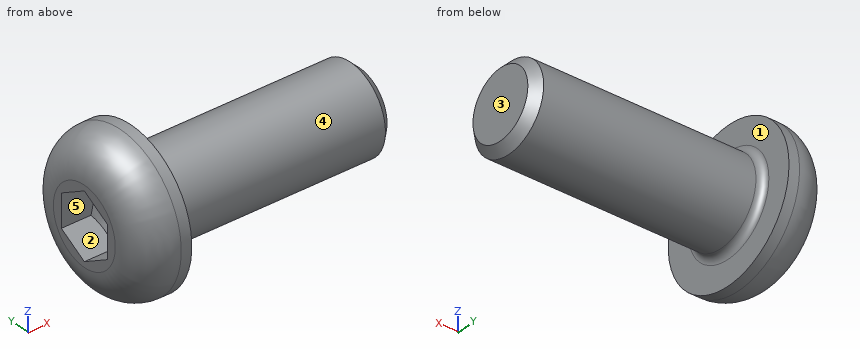
Autodesk Inventor part; units mm, degrees
ref_plane "Work Plane1" through (29, 0, 0) normal (0, -1, 0) x (1, 0, 0)
ref_plane "YZ Plane" through (0, 0, 0) normal (1, 0, 0) x (0, 1, 0)
ref_plane "XZ Plane" through (0, 0, 0) normal (0, 1, 0) x (-1, 0, 0)
sketch "Sketch1" plane through (0, 0, 0) normal (0, 0, 1) x (1, 0, 0)
  line L0 (0.1133, 0) -> (16, 0)
  line L1 (16, 0) -> (16, 3)
  line L2 (16, 3) -> (3, 3)
  line L3 (3, 3) -> (2.3864, 3)
  line L4 (2.3864, 3) -> (0, 3)
  line L5 (0, 3) -> (0, 5.25)
  line L6 (0, 5.25) -> (-3.3, 5.25)
  line L7 (-3.3, 5.25) -> (-3.3, 2.3094)
  line L8 (-3.3, 2.3094) -> (-1.22, 2.3094)
  line L9 (-1.22, 2.3094) -> (0.1133, 0)
  line L10 (-7.16, 0) -> (19.86, 0)
  line L11 (0, -1.05) -> (0, 6.3)
  line L12 (3, 3) -> (0, 3) construction
  dimension "d1" = 13
  dimension "d2" = 0.6136
  dimension "d3" = 3.3
  dimension "d4" = 2.08
  dimension "d5" = 60
  dimension "d6" = 6
  dimension "d7" = 6
  dimension "d8" = 4.6188
  dimension "d9" = 10.5
  dimension "d26" = 16
revolve "Body" add sketch "Sketch1" angle 360 about axis through (0.1133, 0, 0) along (1, 0, 0) contours L9 L11 L4 L3 L2 L1 L0 | L9 L8 L7 L6 L5 L11
sketch "Sketch2" plane through (-3.3, 0, 0) normal (-1, 0, 0) x (0, 0, 1)
  circle A0 centre (0, 0) radius 2.3094
  line L0 (0, -7.35) -> (0, 7.35)
  line L1 (-7.35, 0) -> (7.35, 0)
  line L2 (2.3094, 0) -> (1.1547, -2)
  line L3 (1.1547, -2) -> (-1.1547, -2)
  line L4 (-1.1547, -2) -> (-2.3094, 0)
  line L5 (-2.3094, 0) -> (-1.1547, 2)
  line L6 (-1.1547, 2) -> (1.1547, 2)
  line L7 (1.1547, 2) -> (2.3094, 0)
extrude "Slot" add sketch "Sketch2" against normal up to next contours L7 A0 | A0 L2 | L6 L0 A0 | A0 L0 L3 | L0 L6 A0 | A0 L3 L0 | L4 A0 | A0 L5
fillet "Fillet1" radius 2.56 1 edges at (-3.3, -5.25, 0)
thread "Thread"
chamfer "Chamfer1" distance 0.6135 distance2 0.6135 1 edges at (16, -3, 0) measured on face at (16, -1.1424, 0.935)
ref_plane "Work Plane1" through (29, 0, 0) normal (0, -1, 0) x (1, 0, 0)
fillet "Fillet2" radius 0.5 1 edges at (0, -3, 0)
equation "\"d1\" = GEL"
equation "\"d3\" = KOH"
equation "\"d4\" = INTI"
equation "\"d6\" = GD"
equation "\"d7\" = BDM"
equation "\"d8\" = 1.1547 * SW"
equation "\"d9\" = KOD"
equation "\"d26\" = NLG"
equation "\"d30\" = R"
equation "\"d17\" = RR"
equation "\"d13\" = GEL"
equation "\"d15\" = -0.5 * SPD + 0.5 * GD"
equation "\"d16\" = GUL"
equation "\"GD\" = NND"
equation "\"NLG\" = 16"
equation "\"GEL\" = 13"
equation "\"KOD\" = 10.5"
equation "\"KOH\" = 3.3"
equation "\"INTI\" = 2.08"
equation "\"GAL\" = 0.61345 * PTC"
equation "\"GUL\" = 0.61345 * PTC"
equation "\"BDM\" = NND"
equation "\"SW\" = 4"
equation "\"RR\" = 2.56"
equation "\"SPD\" = NND - 1.2269 * PTC"
equation "\"R\" = 0.5"
equation "\"TOA\" = 30deg"
equation "\"GD1\" = THREADDIA - 1.2269 * PTC"
equation "\"THREADDIA\" = 6"
equation "\"PTC\" = 1"
equation "\"NND\" = 6"
equation "\"KOH1\" = 0.74"
equation "\"E0\" = 4.583"
properties part number "ISO 7380-1 - M6 x 16" material "Steel"
Read the model definition and answer for the solid it produces. Units are mm, in the model's axes. Face numbers are marked on the shaded views. A direction names the side the tool comes from. Give positions to 0.01 mm unless a question says otherwise; leave off trailing zeros. Write each loop counter-clockwise with the first axis right and the second up, starting at its lowest first coordinate (ties: lowest second). Pieces come first, ordered by that corner, then holes. Notation, with made-up numbers: (-33.75, 7) - (-29.75, 7) arc R23 ccw to (-29.75, 45) - close; hole circle Ø9 at (68, -22). An arc over 180 degrees is marked (long way). Answer in a Markdown table with one row per item. Add a question column.
Item 1: Find the intervals of material crossed by L1, parallel to X at y = -1, z = -3.75; L2, parallel to Z at x = 5.5, y = -1; L3, parallel to Y at x = 12.5, z = 2.5, in increasing order.
Item 2: Section A-A, the plane x = 4.25 is taken. Write down the section's boundary in (y, z).
Item 3: Flat-ended cylindrical pins translate along their axes: P1, Ø5, axis at y = 1.5, z = -2.5, coming from the -X side; P2, Ø1.8, axis at x = -2.5, z = 0, coming from the +Y side; P3, Ø3, axis at x = 6.5, z = -2.5, coming from the -Y side; P4, Ø0.7, axis at x = -2, z = 0, coming from the -Y side. Find the tip coordinate at first contact, or state that the pin passes through.
Item 4: A tool of negligible diameter and unlimited length cuts with its end or side. For the marked faces 1 and 2, from which of +Z, -Z, +X, -X, +Y, -Y can it reach the whole face along a straight path? Write none if from no direction.
Item 5: Determine the mould class of the marked faces 3, 4 and 5 for opening direction Z: pulls with the +Z half, pulls with the -Z half, needs draft (parallel to the pull), parting line crosses it, or undercut.
Recorded:
| question | item | result |
|---|---|---|
| 1 | L1 | x = -3.01 to 0 |
| 1 | L2 | z = -2.83 to 2.83 |
| 1 | L3 | y = -1.66 to 1.66 |
| 2 | outline | circle Ø6 at (0, 0) |
| 3 | P1 | stops at x = -3.3 |
| 3 | P2 | stops at y = 5.1 |
| 3 | P3 | stops at y = -2.83 |
| 3 | P4 | stops at y = -5.08 |
| 4 | face 1 | +X |
| 4 | face 2 | -X |
| 5 | face 3 | needs draft |
| 5 | face 4 | parting line crosses it |
| 5 | face 5 | undercut |
